The listing builds one solid part. Answer for the finished solid, in the listing's coordinates (mm). A direction names the side the tool comes from. Coordinates: 2 decimals unless noted, no trailing zeros. Loops run counter-clockwise (first coordinate to the right, second up) from the corner with the lowest first, then second, coordinate; pieces in that order, holes last. Notation, with made-up numbers: M 50,87.25 L 99,87.25 A19 ccw 99,123.25 Z; hole C 16.5,85 d8. An arc over 180 degrees is marked long. Answer as a JSON object with one key per item and string values. Group by question number.
1. A cutting plane is placed at B-B on x = 7. Give the vertices of the cut face in (y, z), and give its area (3 significant figures).
2. Determine the mould class of faces 1 (the face through (-1.5, 11.4, 5.9)), 2 (the face through (-4, 15, 12)), 3 (the face through (0.303, 15.633, 2.673)) for opening direction Y: released by +Y, released by -Y, zero draft, split by the parting line, or undercut.
3. A cutting plane is placed at C-C on y = 0. State how many separate pieces and enclosed holes the cut face has, and give its area (3 significant figures).
4. Given pin 1 (3 mm diameter, centred on y = 9.5, z = -1, fed in from +X); pin 2 (4 mm diameter, centred on x = -7, z = 0.5, fed in from -Y); pin 3 (0.8 mm diameter, centred on x = -0.5, y = 16.5, fed in from -Z), each flat-ended and moving along its own axis, determine where each tip first touches the part or whether it passes through.
5. Straight lines are drawn through the part: L1, parallel to Y at x = 0, z = 4.75; L2, parallel to Y at x = 0, z = 11.5; L3, parallel to Y at x = 0, z = 6.75. For each, find the intervals that lie inside material, in ascending order.
6. A cutting plane is placed at A-A on z = 9. Give the vertices of the cut face in (x, y), and give its area (3 significant figures).
7. For faces 4 (the face through (-5.7, 11.3, 10.5)), 5 (the face through (4, -11, 0)), determine the directions among +Z, -Z, +X, -X, +Y, -Y from which every point of the face is accessible in a straight line to the end or side of a thin tool.
from build123d import *

# Parameters (mm, degrees)
SKETCH1_R           = 19.5
SKETCH1_R_2         = 11.5
EXTRUDE_THIN1_DEPTH = 12
SKETCH2_R           = 1.4
CUT_EXTRUDE1_DEPTH  = 7
CIRPATTERN1_COUNT   = 4
SKETCH5_R           = 15.1
SKETCH5_R_2         = 12.5
CUT_EXTRUDE3_DEPTH  = 1.5
SKETCH6_R           = 1.4
CUT_EXTRUDE4_DEPTH  = 7
CUT_EXTRUDE5_START  = -1.5
SKETCH7_R           = 15.1
SKETCH7_R_2         = 12.5
CUT_EXTRUDE5_DEPTH  = 1.5
EXTRUDE_THIN3_START = 8
SKETCH9_R           = 19.5
SKETCH9_R_2         = 18.5
EXTRUDE_THIN3_DEPTH = 8


with BuildPart() as part:
    # Sketch1 → Extrude-Thin1 (new body)
    with BuildSketch(Plane.XY):
        Circle(SKETCH1_R)
        Circle(SKETCH1_R_2, mode=Mode.SUBTRACT)
    extrude(amount=EXTRUDE_THIN1_DEPTH)

    # Sketch2 → Cut-Extrude1 (cut)
    with BuildSketch(Plane.XY.offset(12)):
        with Locations((0, 17.5)):
            Circle(SKETCH2_R)
    cut_extrude1 = extrude(amount=-CUT_EXTRUDE1_DEPTH, mode=Mode.SUBTRACT)

    # CirPattern1: Cut-Extrude1 ×4 about axis
    cirpattern1_axis = Axis((0, 0, 0), (0, 0, 1))
    for i in range(1, CIRPATTERN1_COUNT):
        add(cut_extrude1.rotate(cirpattern1_axis, i * 360 / CIRPATTERN1_COUNT), mode=Mode.SUBTRACT)

    # Sketch5 → Cut-Extrude3 (cut)
    with BuildSketch(Plane.XY.offset(12)):
        Circle(SKETCH5_R)
        Circle(SKETCH5_R_2, mode=Mode.SUBTRACT)
    extrude(amount=-CUT_EXTRUDE3_DEPTH, mode=Mode.SUBTRACT)

    # Sketch6 → Cut-Extrude4 (cut)
    with BuildSketch(Plane(origin=(0, 0, 0), x_dir=(-1, 0, 0), z_dir=(0, 0, -1))):
        with Locations((0, -17)):
            Circle(SKETCH6_R)
        with Locations((-17, 0)):
            Circle(SKETCH6_R)
        with Locations((0, 17)):
            Circle(SKETCH6_R)
        with Locations((17, 0)):
            Circle(SKETCH6_R)
    extrude(amount=-CUT_EXTRUDE4_DEPTH, mode=Mode.SUBTRACT)

    # Sketch7 → Cut-Extrude5 (cut)
    with BuildSketch(Plane(origin=(0, 0, 0), x_dir=(-1, 0, 0), z_dir=(0, 0, -1)).offset(CUT_EXTRUDE5_START)):
        with Locations(Location((0, 0, 0), (0, 0, 180))):
            Circle(SKETCH7_R)
        with Locations(Location((0, 0, 0), (0, 0, 180))):
            Circle(SKETCH7_R_2, mode=Mode.SUBTRACT)
    extrude(amount=CUT_EXTRUDE5_DEPTH, mode=Mode.SUBTRACT)

    # Sketch9 → Extrude-Thin3 (add)
    with BuildSketch(Plane(origin=(0, 0, 0), x_dir=(-1, 0, 0), z_dir=(0, 0, -1)).offset(EXTRUDE_THIN3_START)):
        Circle(SKETCH9_R)
        Circle(SKETCH9_R_2, mode=Mode.SUBTRACT)
    extrude(amount=-EXTRUDE_THIN3_DEPTH)


solid = part.part
From the geometry:
{
 "1": {"outline": "M -18.2,-8 L -17.12,-8 L -17.12,0 L -13.38,0 L -13.38,1.5 L -10.36,1.5 L -10.36,0 L -9.12,0 L -9.12,12 L -10.36,12 L -10.36,10.5 L -13.38,10.5 L -13.38,12 L -18.2,12 Z; M 9.12,0 L 10.36,0 L 10.36,1.5 L 13.38,1.5 L 13.38,0 L 17.12,0 L 17.12,-8 L 18.2,-8 L 18.2,12 L 13.38,12 L 13.38,10.5 L 10.36,10.5 L 10.36,12 L 9.12,12 Z", "area": "217 mm²"},
 "2": {"face 1": "undercut", "face 2": "zero draft", "face 3": "undercut"},
 "3": {"separate pieces": "4", "enclosed holes": "0", "area": "123 mm²"},
 "4": {"pin 1": "stops at x = 17.78", "pin 2": "stops at y = -18.85", "pin 3": "stops at z = 7"},
 "5": {"L1": "y = -19.5 to -18.4, -15.6 to -11.5, 11.5 to 15.6, 18.4 to 19.5", "L2": "y = -19.5 to -18.9, -16.1 to -15.1, -12.5 to -11.5, 11.5 to 12.5, 15.1 to 16.1, 18.9 to 19.5", "L3": "y = -19.5 to -18.9, -15.6 to -11.5, 11.5 to 15.6, 18.9 to 19.5"},
 "6": {"outline": "C 0,0 d39; hole C -17.5,0 d2.8; hole C 0,0 d23; hole C 0,-17.5 d2.8; hole C 0,17.5 d2.8; hole C 17.5,0 d2.8", "area": "754 mm²"},
 "7": {"face 4": "+Z", "face 5": "-Z"}
}
